from build123d import *

# Parameters (mm, degrees)
F0_R     = 15.5
F1_DEPTH = 40
F2_R     = 15
F3_DEPTH = 40


# Not quite as in the source:
# - a fillet or chamfer that OpenCascade refuses, or shapes differently, is made with other operations: its cross-section is extruded or revolved along the edge and cut away or added


with BuildPart() as f1:
    # F0 (on Front) → F1 (new body)
    with BuildSketch(Plane.XZ):
        Circle(F0_R)
    extrude(amount=F1_DEPTH)

    # F2 (on face) → F3 (cut)
    with BuildSketch(Plane.XZ.offset(40)):
        Circle(F2_R)
    extrude(amount=-F3_DEPTH, mode=Mode.SUBTRACT)

    # F4: fillet of radius 6 on 1 edges, made by hand

    # F4_s1 → F4_t2 (revolve, cut)
    with BuildSketch(Plane.XY):
        with BuildLine():
            ThreePointArc((15.5, -37.6020842383), (15.3736700622, -38.8268291097), (15, -40))
            Line((15, -40), (15.5, -40))
            Line((15.5, -40), (15.5, -37.6020842383))
        make_face()
    revolve(axis=Axis((0, -40, 0), (0, -1, 0)), mode=Mode.SUBTRACT)

    # F5: fillet of radius 6 on 1 edges, made by hand

    # F5_s1 → F5_t2 (revolve, cut)
    with BuildSketch(Plane.XY):
        with BuildLine():
            ThreePointArc((15.5, -2.3979157617), (15.3736700622, -1.1731708903), (15, 0))
            Line((15, 0), (15.5, 0))
            Line((15.5, 0), (15.5, -2.3979157617))
        make_face()
    revolve(axis=Axis((0, 0, 0), (0, -1, 0)), mode=Mode.SUBTRACT)


solid = f1.part
The listing builds one solid part. Answer for the finished solid, in the listing's coordinates (mm). Give positions to 0.01 mm unless a question says otherwise; leave off trailing zeros. Write each loop counter-clockwise with the first axis right and the second up, starting at its lowest first coordinate (ties: lowest second). Pieces come first, ordered by that corner, then holes.
1) Section B-B (z = 0) is taken. Write down the section's boundary in (x, y), and give its area (3 significant figures).
2) Find the intervals of material crossed by L1, parallel to Z at x = 0, y = -31; L2, parallel to X at y = -17, z = -6.5; L3, parallel to Z at x = -4.5, y = -2, in increasing order.
3) For a pull along X with two mould halves and no side action, classify faces 1 (the face through (-2.018, -19.754, 15.368)), 2 (the face through (-14.985, -20.28, 0.66)) as pulls with the +X half, pulls with the -X half, needs draft (parallel to the pull), parting line crosses it, or undercut.
4) Section A-A (x = 0) is taken. Write down the section's boundary in (y, z).
5) Given P1, Ø12, axis at x = 9, y = -14.5, coming from the -Z side; P2, Ø12, axis at x = -8, y = -16.5, coming from the +Z side; P3, Ø12, axis at x = 4, z = -11.5, coming from the +Y side; P4, Ø3, axis at x = -8, y = -5, coming from the -Z side, each flat-ended and moving along its own axis, determine where each tip first touches the part or whether it passes through.
6) Section C-C (y = -14) is taken. Write down the section's boundary in (x, z).
Response:
1. outline: (-15.5, -37.6) arc R6 ccw to (-15, -40) - (-15, 0) arc R6 ccw to (-15.5, -2.4) - close; (15, -40) arc R6 ccw to (15.5, -37.6) - (15.5, -2.4) arc R6 ccw to (15, 0) - close
1. area: 38.4 mm2
2. L1: z = -15.5 to -15, 15 to 15.5
2. L2: x = -14.07 to -13.52, 13.52 to 14.07
2. L3: z = -14.82 to -14.31, 14.31 to 14.82
3. face 1: parting line crosses it
3. face 2: undercut
4. outline: (-40, -15) arc R6 ccw to (-37.6, -15.5) - (-2.4, -15.5) arc R6 ccw to (0, -15) - close; (-40, 15) - (0, 15) arc R6 ccw to (-2.4, 15.5) - (-37.6, 15.5) arc R6 ccw to start
5. P1: stops at z = -15.21
5. P2: stops at z = 15.37
5. P3: stops at y = 0
5. P4: stops at z = -14.07
6. outline: circle Ø31 at (0, 0); hole circle Ø30 at (0, 0)
